Geometry: final body of the model. Coordinates: model frame, mm. Face numbers are marked on the shaded views. A direction names the side the tool comes from. Coordinates: 2 decimals unless noted, no trailing zeros. Order: outer loops, then holes, each group sorted by start corner. A loop starts at its lowest first (then second) coordinate and runs counter-clockwise, first axis right, second up. Notation, with made-up numbers: (-25, 49) -> (-8, 49) arc R29 cw to (-8, 71) -> close; hole circle Ø6 at (14, 36). An arc over 180 degrees is marked (long way). Use CSV: the item, a comma, the result in double quotes. Start each with the question number.
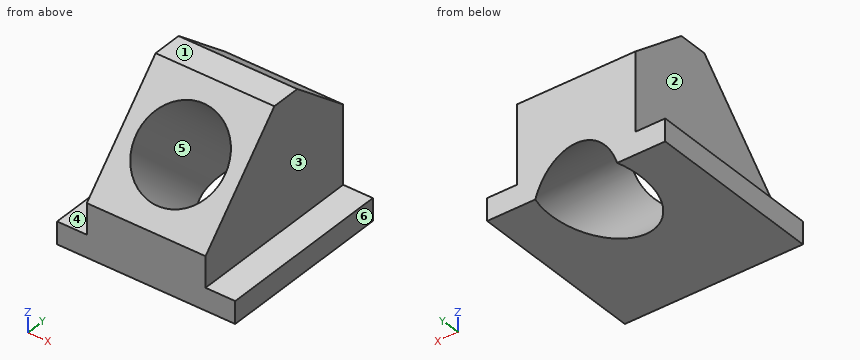
from build123d import *

# Parameters (mm, degrees)
F0_W     = 12.773345685
F0_H     = 76.2
F0_W_2   = 12.626654315
F0_W_3   = 50.8
F1_DEPTH = 9.525
F2_W     = 50.8
F2_H     = 76.2
F3_DEPTH = 63.5
F5_DEPTH = 107.696
F6_R     = 19.05
F7_DEPTH = 89.662


with BuildPart() as f1:
    # F0 (on Top) → F1 (new body)
    with BuildSketch(Plane.XY):
        with Locations((-31.2884969145, -3.5850352719)):
            Rectangle(F0_W, F0_H)
        with Locations((32.2115030855, -3.5850352719)):
            Rectangle(F0_W_2, F0_H)
        with Locations((0.498175928, -3.5850352719)):
            Rectangle(F0_W_3, F0_H)
    extrude(amount=F1_DEPTH)

    # F2 (on face) → F3 (join)
    with BuildSketch(Plane(origin=(0, 0, 0), x_dir=(1, 0, 0), z_dir=(0, 0, -1))):
        with Locations((0.424830243, 3.5850352719)):
            Rectangle(F2_W, F2_H)
    extrude(amount=-F3_DEPTH)

    # F4 (on face) → F5 (cut)
    with BuildSketch(Plane(origin=(-24.975169757, 0, 0), x_dir=(0, -1, 0), z_dir=(-1, 0, 0))):
        Polygon((-34.5149647281, 63.5), (-34.5149647281, 42.8782887757), (-9.1149647281, 63.5), align=None)
        Polygon((41.6850352719, 63.5), (3.5850352719, 63.5), (41.6850352719, 22.6427521481), align=None)
    extrude(amount=-F5_DEPTH, mode=Mode.SUBTRACT)

    # F6 (on face) → F7 (cut)
    with BuildSketch(Plane(origin=(0, -33.5902159411, 31.3233831117), x_dir=(1, 0, 0), z_dir=(0, -0.7313537016, 0.6819983601))):
        with Locations((0.424830243, 16.0633533902)):
            Circle(F6_R)
    extrude(amount=-F7_DEPTH, mode=Mode.SUBTRACT)


solid = f1.part
(1) Mould query, pull axis Z, two halves, no side actions, for the marked faces 4, 5 and 6. Classes: pulls with the +Z half, pulls with the -Z half, needs draft (parallel to the pull), parting line crosses it, or undercut.
(2) Section A-A (x = 16.5). Return loops of the section in (y, z).
(3) Line query: line 1 (X direction, y = -30.5, z = 11); line 2 (Z direction, x = -30, y = -29.5) (3 decimals); line 3 (X direction, y = -3, z = 36). Output: solid intervals per line, ascending. Write a range as from..to.
(4) Access query for the marked faces 1, 2 and 3. Directions: +Z, -Z, +X, -X, +Y, -Y. A direction counts if a zero-diameter tool reaches every point of the face in a straight line with its end or side. Return the directions, or none.
(5) First-contact query: pin 1 (1 mm diameter, centred on x = -6.5, y = -7, fed in from +Z); pin 2 (12 mm diameter, centred on x = 7, y = 11.5, fed in from -Z); pin 3 (8 mm diameter, centred on y = 23.5, z = 46.5, fed in from +X). Flat tips, straight axial feed; report the tip coordinate or a pass-through.
(6) Section B-B (z = 60.5). Return loops of the section in (x, y).
Check sheet entries:
1,face 4,"pulls with the +Z half"
1,face 5,"undercut"
1,face 6,"needs draft"
2,outline,"(-41.69, 0) -> (8.56, 0) -> (-29.61, 35.6) -> (-41.69, 22.64) -> close; (-15.66, 50.55) -> (34.51, 3.76) -> (34.51, 42.88) -> (9.11, 63.5) -> (-3.59, 63.5) -> close"
3,line 1,"x = -24.98..25.82"
3,line 2,"z = 0..9.525"
3,line 3,"x = -24.98..-16.76, 17.61..25.82"
4,face 1,"+Z, +X, -X, +Y, -Y"
4,face 2,"+Z, -X, +Y, -Y"
4,face 3,"+Z, +X, +Y, -Y"
5,pin 1,"stops at z = 60.37"
5,pin 2,"stops at z = 28.72"
5,pin 3,"stops at x = 25.82"
6,outline,"(-24.98, -6.38) -> (25.82, -6.38) -> (25.82, 12.81) -> (-24.98, 12.81) -> close"
